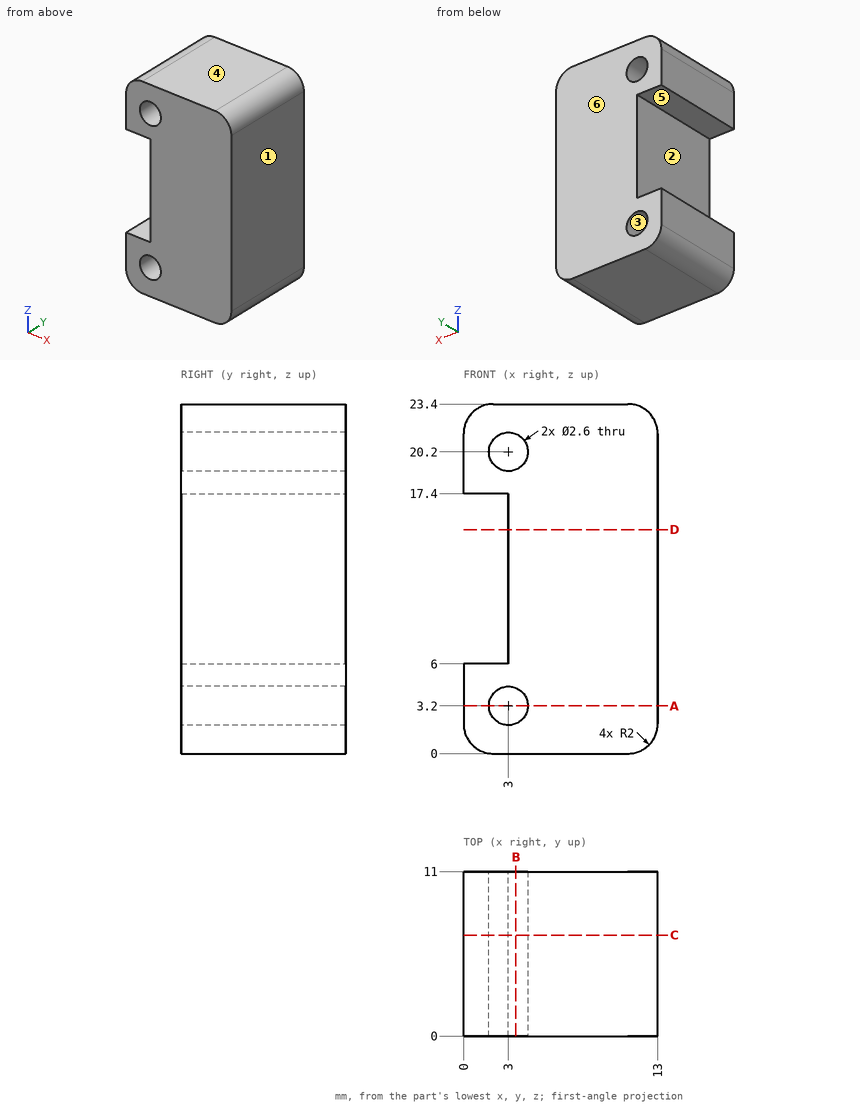
Could you check a few things on this drawing? It's one solid part, dimensions in mm from its lowest x, y, z. A direction names the side the tool comes from. Round coordinates to 2 decimals unless told otherwise and drop trailing zeros. Loops run counter-clockwise (first coordinate to the right, second up) from the corner with the lowest first, then second, coordinate; pieces in that order, holes last. Notation, with made-up numbers: M -35,-27 L -5,-27 A20 ccw -5,-22 Z; hole C 45,-37 d3. An arc over 180 degrees is marked long. Write item = value, one per line. Start each with the question number.
(1) Which directions (+Z, -Z, +X, -X, +Y, -Y) give clear straight access to the entire face, cutting with the end or side of a thin tool? Please do the marked faces 5 and 6.
(2) If we mould it in two halves opening along Z, with no side actions, what happens to the marked faces 1, 2, 3 and 4? For each: released by +Z, released by -Z, zero draft, split by the parting line, or undercut.
(3) Suppose I cut it at A-A on z = 3.2. Write out the boundary of the cut face in (x, y).
(4) Suppose I cut it at D-D on z = 15. Write out the boundary of the cut face in (x, y), plus the area to 3 significant figures.
(5) I need wall thicknesses on line 1 along Z through (x, y) = (2.75, 3.5); line 2 along Z through (x, y) = (3.75, 1); line 3 along X through (y, z) = (6.25, 11.75). Which ranges of each line are inside material? Lowest first, please.
(6) I'm going to push flat-ended pins straight in: P1, Ø5.5, axis at y = 4, z = 14, coming from the -X side; P2, Ø3, axis at x = 3, z = 3.2, coming from the +Y side; P3, Ø1.5, axis at x = 1, y = 7.5, coming from the +Z side. Where does each tip first touch, or does it pass through?
(7) Suppose I cut it at C-C on y = 6.75. Write out the boundary of the cut face in (x, z), plus the area to 3 significant figures.
(8) Suppose I cut it at B-B on x = 3.5. Write out the boundary of the cut face in (y, z).
Answer block:
q1.face_5 = -X, +Y, -Y
q1.face_6 = +Z, -Z, +X, -X, +Y
q2.face_1 = zero draft
q2.face_2 = undercut
q2.face_3 = undercut
q2.face_4 = released by +Z
q3.outline = M 0,0 L 1.7,0 L 1.7,11 L 0,11 Z; M 4.3,0 L 13,0 L 13,11 L 4.3,11 Z
q4.outline = M 3,0 L 13,0 L 13,11 L 3,11 Z
q4.area = 110 mm²
q5.line_1 = 0 to 1.92, 4.48 to 6, 17.4 to 18.92, 21.48 to 23.4
q5.line_2 = 0 to 2.14, 4.26 to 19.14, 21.26 to 23.4
q5.line_3 = 3 to 13
q6.P1 = 3
q6.P2 = 11
q6.P3 = 23.38
q7.outline = M 0,2 A2 ccw 2,0 L 11,0 A2 ccw 13,2 L 13,21.4 A2 ccw 11,23.4 L 2,23.4 A2 ccw 0,21.4 L 0,17.4 L 3,17.4 L 3,6 L 0,6 Z; hole C 3,3.2 d2.6; hole C 3,20.2 d2.6
q7.area = 256 mm²
q8.outline = M 0,0 L 11,0 L 11,2 L 0,2 Z; M 0,4.4 L 11,4.4 L 11,19 L 0,19 Z; M 0,21.4 L 11,21.4 L 11,23.4 L 0,23.4 Z
